Could you check a few things on this drawing? It's one solid part, dimensions in mm from its lowest x, y, z. Give positions to 0.01 mm unless a question says otherwise; leave off trailing zeros. Order: outer loops, then holes, each group sorted by start corner. A loop starts at its lowest first (then second) coordinate and runs counter-clockwise, first axis right, second up. Notation, with made-up numbers: M 35.5,59 L 90.5,59 A34 cw 90.5,97 Z; hole C 49,56 d10. An arc over 180 degrees is marked long. Use one line per item in the form item = value. Start each with the question number.
1. I want a section at A-A, the plane z = 10. List the corners of the cut face in (x, y) for me.
2. I need wall thicknesses on L1, parallel to Y at x = 5, z = 7.75; L2, parallel to Y at x = 12.5, z = 11.25; L3, parallel to X at y = 11.75, z = 6.75 (1 decimal). Which ranges of each line are inside material? Lowest first, please.
3. I want a section at C-C, the plane x = 10. List the corners of the cut face in (y, z) for me.
4. I want a section at B-B, the plane y = 6.35. List the corners of the cut face in (x, z) for me, and give its area (3 significant figures).
5. Will these pins go through, and if not, where does the flat tip stop? P1, Ø4, axis at x = 21.5, y = 9.5, coming from the -Z side (1 decimal); P2, Ø1, axis at y = 7.5, z = 10, coming from the +X side (1 decimal); P3, Ø1, axis at x = 34, z = 4.5, coming from the +Y side (1 decimal).
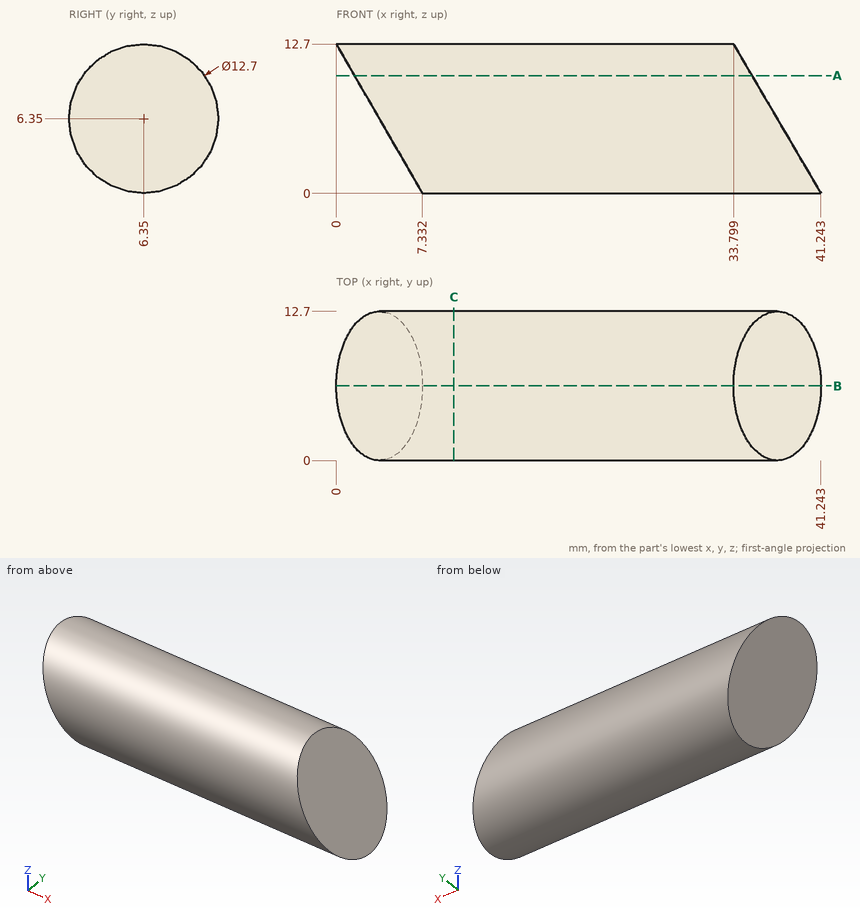
Check result:
q1.outline = M 1.56,1.15 L 35.38,1.15 L 35.38,11.55 L 1.56,11.55 Z
q2.L1 = 0.16 to 12.54
q2.L2 = 2.31 to 10.39
q2.L3 = 3.4 to 37.3
q3.outline = C 6.35,6.35 d12.7
q4.outline = M 0,12.7 L 7.33,0 L 41.24,0 L 33.8,12.7 Z
q4.area = 430 mm2
q5.P1 = 0.1
q5.P2 = 35.7
q5.P3 = 12.6
